Can you work these out from the model? Positions are in its coordinate system, mm. Face numbers are marked on the shaded views. A direction names the side the tool comes from. Coordinates: 2 decimals unless noted, no trailing zeros. Order: outer loops, then holes, each group sorted by start corner. A loop starts at its lowest first (then second) coordinate and runs counter-clockwise, first axis right, second up. Notation, with made-up numbers: (9, 75) -> (35, 75) arc R23 ccw to (35, 90) -> close; hole circle Ø6 at (87.5, -5). An arc over 180 degrees is marked (long way). Answer as a JSON object with one key per item and string values. Group by question number.
(1) For pin 1 (17 mm diameter, centred on x = 25.85, z = -25.85, fed in from +Y); pin 2 (1.9 mm diameter, centred on y = 9.5, z = -46.5, fed in from +X); pin 3 (5 mm diameter, centred on y = 12, z = -43.5, fed in from -X), each with a flat end and sliding along its axis, tell me the tip position at first contact or that it passes through.
(2) I want a section at D-D, the plane y = 31.5. List the corners of the cut face in (x, z) for me.
(3) I want a section at B-B, the plane z = 0. List the corners of the cut face in (x, y) for me.
(4) Which directions (+Z, -Z, +X, -X, +Y, -Y) give clear straight access to the entire face, cutting with the end or side of a thin tool? Please do the marked faces 4 and 5.
(5) I need wall thicknesses on line 1 (X direction, y = 5.5, z = 0); line 2 (X direction, y = 16, z = 0); line 3 (X direction, y = 9.5, z = -6.5). Which ranges of each line are inside material? Lowest first, please.
(6) I want a section at C-C, the plane z = 12. List the corners of the cut face in (x, y) for me, plus the area to 3 significant figures.
(7) If we mould it in two halves opening along Z, with no side actions, what happens to the marked faces 1, 2 and 3? For each: pulls with the +Z half, pulls with the -Z half, needs draft (parallel to the pull), parting line crosses it, or undercut.
(8) I want a section at A-A, the plane x = 0. List the corners of the cut face in (y, z) for me.
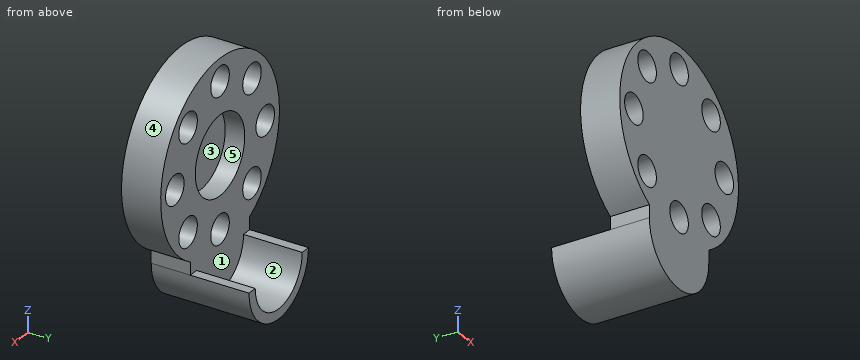
from build123d import *

# Parameters (mm, degrees)
EXTRUDE_1_DEPTH     = 20
SKETCH_2_R          = 20
CUT_EXTRUDE_1_DEPTH = 10
SKETCH_3_R          = 7.5
CUT_EXTRUDE_2_DEPTH = 89.814413245
EXTRUDE_2_DEPTH     = 30


with BuildPart() as part:
    # 草圖1 → 填料-伸長1 (new body)
    with BuildSketch(Plane(origin=(0, 0, 0), x_dir=(1, 0, 0), z_dir=(0, 1, 0))):
        with BuildLine():
            Line((-24, 41.569219382), (-24, 48))
            ThreePointArc((-24, 48), (0, 72), (24, 48))
            Line((24, 48), (24, 41.569219382))
            ThreePointArc((24, 41.569219382), (0, -48), (-24, 41.569219382))
        make_face()
    extrude(amount=EXTRUDE_1_DEPTH)

    # 草圖2 → 除料-伸長1 (cut)
    with BuildSketch(Plane(origin=(0, 20, 0), x_dir=(1, 0, 0), z_dir=(0, 1, 0))):
        with Locations(Location((0, 0, 0), (0, 0, 270))):
            Circle(SKETCH_2_R)
    extrude(amount=-CUT_EXTRUDE_1_DEPTH, mode=Mode.SUBTRACT)

    # 草圖3 → 除料-伸長2 (cut, through all)
    with BuildSketch(Plane(origin=(0, 20, 0), x_dir=(1, 0, 0), z_dir=(0, 1, 0))):
        with Locations(Location((0, 36.553135894, 0), (0, 0, 270))):
            Circle(SKETCH_3_R)
        with Locations(Location((25.846970264, 25.846970264, 0), (0, 0, 270))):
            Circle(SKETCH_3_R)
        with Locations(Location((36.553135894, 0, 0), (0, 0, 270))):
            Circle(SKETCH_3_R)
        with Locations(Location((25.846970264, -25.846970264, 0), (0, 0, 270))):
            Circle(SKETCH_3_R)
        with Locations(Location((0, -36.553135894, 0), (0, 0, 270))):
            Circle(SKETCH_3_R)
        with Locations(Location((-25.846970264, -25.846970264, 0), (0, 0, 270))):
            Circle(SKETCH_3_R)
        with Locations(Location((-36.553135894, 0, 0), (0, 0, 270))):
            Circle(SKETCH_3_R)
        with Locations(Location((-25.846970264, 25.846970264, 0), (0, 0, 270))):
            Circle(SKETCH_3_R)
    extrude(amount=-CUT_EXTRUDE_2_DEPTH, mode=Mode.SUBTRACT)

    # 草圖4 → 填料-伸長2 (add)
    with BuildSketch(Plane(origin=(0, 20, 0), x_dir=(1, 0, 0), z_dir=(0, 1, 0))):
        with BuildLine():
            Line((-24, 48), (-19, 48))
            ThreePointArc((-19, 48), (0, 67), (19, 48))
            Line((19, 48), (24, 48))
            ThreePointArc((24, 48), (0, 72), (-24, 48))
        make_face()
    extrude(amount=EXTRUDE_2_DEPTH)


solid = part.part
Computed values:
{
 "1": {"pin 1": "stops at y = 20", "pin 2": "stops at x = 24", "pin 3": "stops at x = -24.96"},
 "2": {"outline": "(-24, -48) arc R24 ccw to (24, -48) -> (19, -48) arc R19 cw to (-19, -48) -> close"},
 "3": {"outline": "(-48, 0) -> (-44.05, 0) -> (-44.05, 20) -> (-48, 20) -> close; (-29.05, 0) -> (29.05, 0) -> (29.05, 20) -> (20, 20) -> (20, 10) -> (-20, 10) -> (-20, 20) -> (-29.05, 20) -> close; (44.05, 0) -> (48, 0) -> (48, 20) -> (44.05, 20) -> close"},
 "4": {"face 4": "+Y, -Y", "face 5": "+Y"},
 "5": {"line 1": "x = -48 to -44.05, -29.05 to 29.05, 44.05 to 48", "line 2": "x = -48 to -44.05, -29.05 to -20, 20 to 29.05, 44.05 to 48", "line 3": "x = -47.56 to -40.29, -32.81 to 32.81, 40.29 to 47.56"},
 "6": {"outline": "(-46.48, 0) -> (46.48, 0) -> (46.48, 20) -> (16, 20) -> (16, 10) -> (-16, 10) -> (-16, 20) -> (-46.48, 20) -> close", "area": "1,540 mm2"},
 "7": {"face 1": "needs draft", "face 2": "pulls with the +Z half", "face 3": "undercut"},
 "8": {"outline": "(0, -72) -> (50, -72) -> (50, -67) -> (20, -67) -> (20, -44.05) -> (0, -44.05) -> close; (0, -29.05) -> (20, -29.05) -> (20, -20) -> (10, -20) -> (10, 20) -> (20, 20) -> (20, 29.05) -> (0, 29.05) -> close; (0, 44.05) -> (20, 44.05) -> (20, 48) -> (0, 48) -> close"}
}
